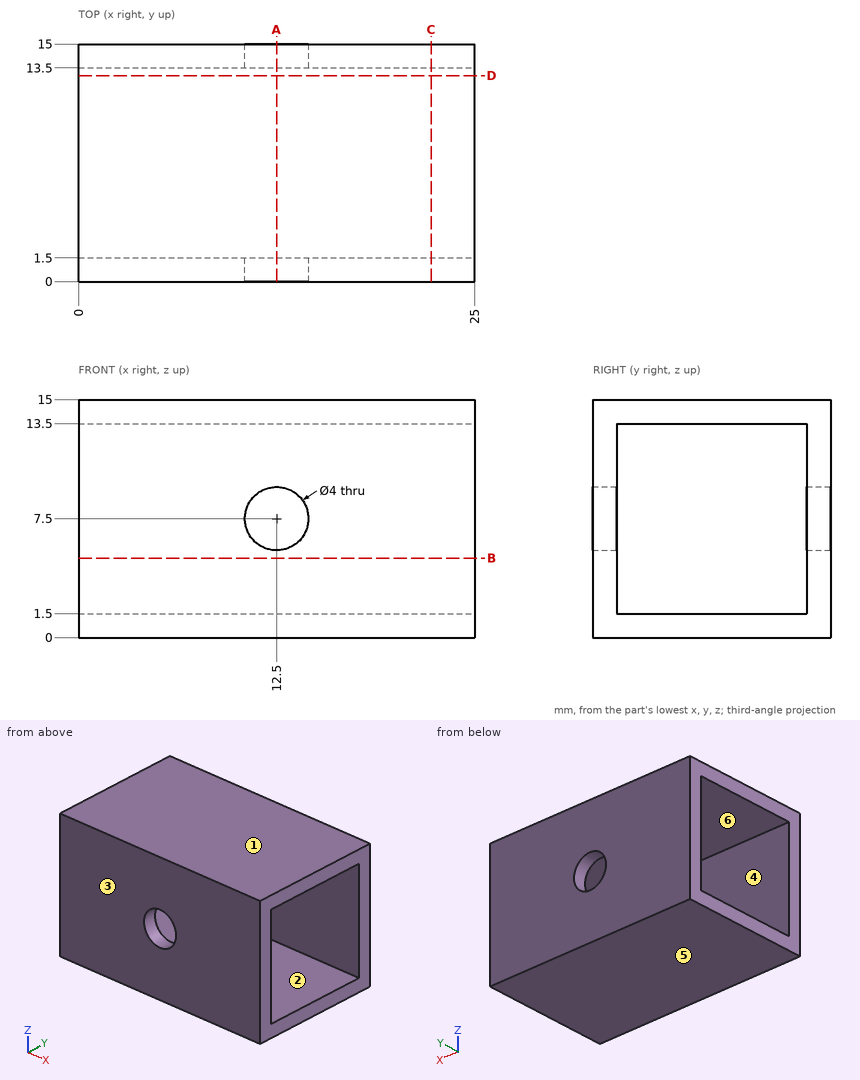
The figure shows three views and two pictorial views of one solid part (mm, origin at its lowest corner). Answer the questions. A direction names the side the tool comes from. Round coordinates to 2 decimals unless told otherwise and drop trailing zeros. Order: outer loops, then holes, each group sorted by start corner. A loop starts at its lowest first (then second) coordinate and runs counter-clockwise, first axis right, second up. Notation, with made-up numbers: M 59,12.25 L 89,12.25 A11 ccw 89,17.25 Z; hole C 58.25,5 d2. An arc over 180 degrees is marked long. Put each result on its own line as item: value. Start each with the question number.
Q1. Section C-C, the plane x = 22.25 is taken. Write down the section's boundary in (y, z).
Q2. Section A-A, the plane x = 12.5 is taken. Write down the section's boundary in (y, z).
Q3. A tool of negligible diameter and unlimited length cuts with its end or side. For the marked faces 1 and 2, from which of +Z, -Z, +X, -X, +Y, -Y can it reach the whole face along a straight path? Write none if from no direction.
Q4. For a pull along Y with two mould halves and no side action, classify the marked faces 3, 4, 5 and 6 as pulls with the +Y half, pulls with the -Y half, needs draft (parallel to the pull), parting line crosses it, or undercut.
Q5. Straight lines are drawn through the part: L1, parallel to Z at x = 12.5, y = 14.35; L2, parallel to Y at x = 14, z = 5. For each, find the intervals that lie inside material, in ascending order. Write a range as [from, to].
Q6. Section B-B, the plane z = 5 is taken. Write down the section's boundary in (x, y).
Q7. A flat-ended cylindrical pin translates along its axis: pin 1 (8 mm diameter, centred on x = 3, z = 5.5, fed in from -Y). Find the tip coordinate at first contact, or state that the pin passes through.
Findings below:
1. outline: M 0,0 L 15,0 L 15,15 L 0,15 Z; hole M 1.5,1.5 L 13.5,1.5 L 13.5,13.5 L 1.5,13.5 Z
2. outline: M 0,0 L 15,0 L 15,5.5 L 13.5,5.5 L 13.5,1.5 L 1.5,1.5 L 1.5,5.5 L 0,5.5 Z; M 0,9.5 L 1.5,9.5 L 1.5,13.5 L 13.5,13.5 L 13.5,9.5 L 15,9.5 L 15,15 L 0,15 Z
3. face 1: +Z, +X, -X, +Y, -Y
3. face 2: +X, -X
4. face 3: pulls with the -Y half
4. face 4: undercut
4. face 5: needs draft
4. face 6: undercut
5. L1: z = [0, 5.5], [9.5, 15]
5. L2: y = [0, 1.5], [13.5, 15]
6. outline: M 0,0 L 25,0 L 25,1.5 L 0,1.5 Z; M 0,13.5 L 25,13.5 L 25,15 L 0,15 Z
7. pin 1: stops at y = 0
